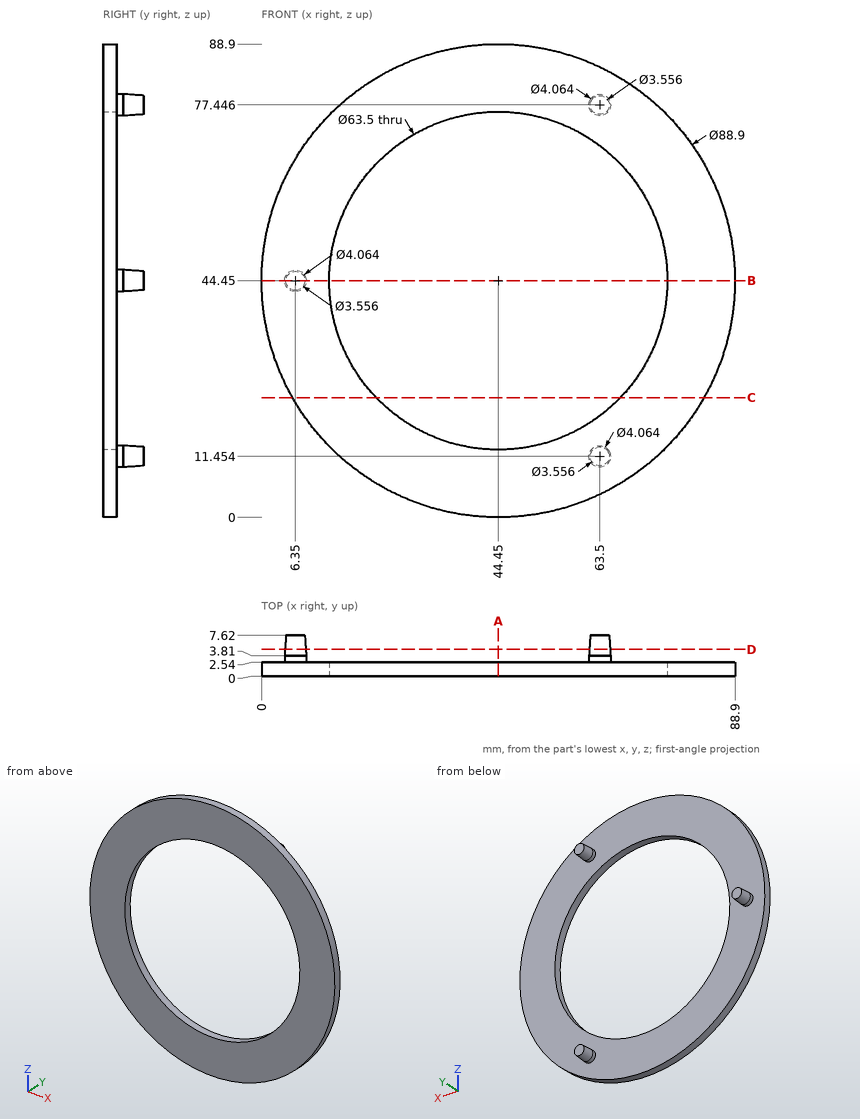
Geometry check sheet. Reference: drawing and pictorial views, mm from the part's lowest x, y, z. Coordinates: 2 decimals unless noted, no trailing zeros. Loops run counter-clockwise (first coordinate to the right, second up) from the corner with the lowest first, then second, coordinate; pieces in that order, holes last.
1) Sectioned sample at D-D (y = 5). Count the separate pieces of the cut face and the enclosed holes in it.
2) Gauge pin test, flat ends, axial feed: pin 1 (5 mm diameter, centred on x = 23.5, z = 17.5, fed in from -Y); pin 2 (3 mm diameter, centred on x = 24, y = 2, fed in from +Z); pin 3 (3 mm diameter, centred on y = 3.5, z = 26, fed in from -X); pin 4 (2 mm diameter, centred on x = 72.5, z = 56, fed in from +Y). Record the tip position at first contact, or that the pin passes through.
3) Sectioned sample at C-C (z = 22.5). Record the boundary of the cut face in (x, y).
4) Sectioned sample at B-B (z = 44.45). Record the boundary of the cut face in (x, y).
5) Sectioned sample at A-A (x = 44.45). Record the boundary of the cut face in (y, z).
6) Material ranges on probe 1 along X at (y, z) = (0.9, 44.45); probe 2 along Y at (x, z) = (60.5, 75); probe 3 along Z at (x, y) = (50.5, 2), recorded low to high.
Check sheet entries:
1. separate pieces: 3
1. enclosed holes: 0
2. pin 1: stops at y = 0
2. pin 2: stops at z = 84.66
2. pin 3: stops at x = 3.5
2. pin 4: passes through
3. outline: (5.8, 0) - (21.51, 0) - (21.51, 2.54) - (5.8, 2.54) - close; (67.39, 0) - (83.1, 0) - (83.1, 2.54) - (67.39, 2.54) - close
4. outline: (0, 0) - (12.7, 0) - (12.7, 2.54) - (8.38, 2.54) - (8.38, 3.81) - (8.13, 7.62) - (4.57, 7.62) - (4.32, 3.81) - (4.32, 2.54) - (0, 2.54) - close; (76.2, 0) - (88.9, 0) - (88.9, 2.54) - (76.2, 2.54) - close
5. outline: (0, 0) - (2.54, 0) - (2.54, 12.7) - (0, 12.7) - close; (0, 76.2) - (2.54, 76.2) - (2.54, 88.9) - (0, 88.9) - close
6. probe 1: x = 0 to 12.7, 76.2 to 88.9
6. probe 2: y = 0 to 2.54
6. probe 3: z = 0.41 to 13.28, 75.62 to 88.49
